For this review, take the finished solid that the model builds, in its own axes (mm). A direction names the side the tool comes from. Coordinates: 2 decimals unless noted, no trailing zeros. Write each loop counter-clockwise with the first axis right and the second up, starting at its lowest first coordinate (ties: lowest second). Pieces come first, ordered by that corner, then holes. Notation, with made-up numbers: (-17.75, 6) - (7.25, 6) arc R4 ccw to (7.25, 13) - close; hole circle Ø10 at (89, -33). An arc over 180 degrees is marked (long way). Write each question's results on one line, items separated by ' | '.
from build123d import *

# Parameters (mm, degrees)
F0_R      = 21.2
F1_DEPTH  = 800
F2_R      = 5
F3_DEPTH  = 50
F4_W      = 150
F4_H      = 100
F5_DEPTH  = 10
F7_D      = 14
F9_DEPTH  = 650
F10_W     = 18.732145
F10_H     = 50
F10_W_2   = 18.157326
F11_DEPTH = 25
F12_W     = 15.213338
F12_H     = 518.766022
F13_DEPTH = 25


with BuildPart() as f1:
    # F0 (on Top) → F1 (new body)
    with BuildSketch(Plane.XY):
        Circle(F0_R)
    extrude(amount=F1_DEPTH)

    # F2 (on face) → F3 (join)
    with BuildSketch(Plane.XY.offset(800)):
        Circle(F2_R)
    extrude(amount=F3_DEPTH)

    # F4 (on face) → F5 (join)
    with BuildSketch(Plane(origin=(0, 0, 0), x_dir=(1, 0, 0), z_dir=(0, 0, -1))):
        Rectangle(F4_W, F4_H)
    extrude(amount=F5_DEPTH)

    # F7 (through all)
    with Locations(Plane(origin=(0, 0, -10), x_dir=(1, 0, 0), z_dir=(0, 0, -1))):
        with Locations((-50, 0), (50, 0)):
            Hole(F7_D / 2)

    # F8 (on face) → F9 (join)
    with BuildSketch(Plane.XY.offset(800)):
        Polygon((36.2, -3), (36.2, 0), (36.2, 3), (20.986662, 3), (20.986662, -3), align=None)
        Polygon((-36.2, 3), (-36.2, 0), (-36.2, -3), (-20.986662, -3), (-20.986662, 3), align=None)
    extrude(amount=-F9_DEPTH)

    # F10 (on face) → F11 (cut)
    with BuildSketch(Plane.XZ.offset(3)):
        with Locations((-30.352734, 775)):
            Rectangle(F10_W, F10_H)
        with Locations((30.178081, 775)):
            Rectangle(F10_W_2, F10_H)
    extrude(amount=-F11_DEPTH, mode=Mode.SUBTRACT)

    # F12 (on face) → F13 (cut)
    with BuildSketch(Plane.XZ.offset(3)):
        with Locations((-28.593331, 450.616989)):
            Rectangle(F12_W, F12_H)
        Polygon((39.251614, 190.913462), (39.251614, 709.418058), (20.16026, 709.418058), (20.16026, 190.913462), (36.762826, 190.913462), align=None)
    extrude(amount=-F13_DEPTH, mode=Mode.SUBTRACT)


solid = f1.part
Q1. For pin 1 (16.5 mm diameter, centred on x = -26, z = 731, fed in from +Y); pin 2 (12.5 mm diameter, centred on x = 8.5, y = -9.5, fed in from +Z); pin 3 (1.5 mm diameter, centred on x = -7, y = 21.5, fed in from +Z), all flat-tipped, find the tip position at first contact; note any pin that passes through.
Results found:
pin 1: y = 11.59 | pin 2: z = 800 | pin 3: z = 0
Q2. Wall thickness on line 1 along Y through (x, z) = (50, -4.5); line 2 along Z through (x, y) = (-47, 30.5); line 3 along Z through (x, y) = (7, 9): over which ranges is each line inside the solid? List them lowest first. Write a range as from..to.
Results found:
line 1: -50..-7, 7..50 | line 2: -10..0 | line 3: -10..800
Q3. For faces 1 (the face through (-28, 3, 730)), 2 (the face through (28, -3, 171)), 3 (the face through (29, 3, 171)), 4 (the face through (-29, -3, 730)), list the 3-axis set-ups (+Z, -Z, +X, -X, +Y, -Y) from which the entire face can be reached by the end or side of a thin tool; tool diameter is ignored.
Results found:
face 1: +Z, -X, +Y | face 2: +Z, +X, -Y | face 3: +Z, +X, +Y | face 4: +Z, -X, -Y
Q4. Take a section at B-B on y = 42.5. State the section outline as (x, z) points, plus the area to 3 significant figures.
Results found:
outline: (-75, -10) - (75, -10) - (75, 0) - (-75, 0) - close | area: 1,500 mm2
Q5. Take a section at A-A on z = 163. State the section outline as (x, y) points, plus the area to 3 significant figures.
Results found:
outline: (-36.2, -3) - (-20.99, -3) arc R21.2 ccw to (20.99, -3) - (36.2, -3) - (36.2, 3) - (20.99, 3) arc R21.2 ccw to (-20.99, 3) - (-36.2, 3) - close | area: 1,590 mm2
